from build123d import *

# Parameters (mm, degrees)
BOSS_EXTRUDE1_DEPTH = 20
BOSS_EXTRUDE2_REACH = 35.797


with BuildPart() as part:
    # Sketch1 → Boss-Extrude1 (new, symmetric)
    with BuildSketch(Plane(origin=(0, 0, 0), x_dir=(0, 0, -1), z_dir=(1, 0, 0))):
        Polygon((-8, 0), (-8, 17.5), (8, 17.5), (8, 0), (10.5, 0), (10.5, 20), (-10.5, 20), (-10.5, 0), align=None)
    extrude(amount=BOSS_EXTRUDE1_DEPTH, both=True)

    # Sketch2 → Boss-Extrude2 (add, up to next)
    with BuildSketch(Plane(origin=(0, 0, 8), x_dir=(-1, 0, 0), z_dir=(0, 0, -1)), mode=Mode.PRIVATE) as boss_extrude2_sk1:
        with BuildLine():
            Line((20, 17.5), (20, 20))
            Line((20, 20), (-20, 20))
            Line((-20, 20), (-20, 17.5))
            ThreePointArc((-20, 17.5), (0, 9.985297678), (20, 17.5))
        make_face()
    boss_extrude2_tool1 = extrude(boss_extrude2_sk1.sketch, amount=BOSS_EXTRUDE2_REACH, mode=Mode.PRIVATE) - part.part
    add(boss_extrude2_tool1.solids().sort_by_distance((0, 15.86208, 8))[0])


solid = part.part
Read the model definition and answer for the solid it produces. Units are mm, in the model's axes. Round coordinates to 2 decimals unless told otherwise and drop trailing zeros. Write each loop counter-clockwise with the first axis right and the second up, starting at its lowest first coordinate (ties: lowest second). Pieces come first, ordered by that corner, then holes.
Q1. Straight lines are drawn through the part: line 1 (Z direction, x = 7.5, y = 2); line 2 (X direction, y = 13.5, z = -6); line 3 (Y direction, x = 10, z = 3). For each, find the intervals that lie inside material, in ascending order.
Values:
line 1: z = -10.5 to -8, 8 to 10.5
line 2: x = -14.18 to 14.18
line 3: y = 11.68 to 20
Q2. Find section D-D on x = 3.5. Determine the outline of the cut face in (y, z), and give its area (3 significant figures).
Values:
outline: (0, -10.5) - (20, -10.5) - (20, 10.5) - (0, 10.5) - (0, 8) - (10.19, 8) - (10.19, -8) - (0, -8) - close
area: 257 mm2
Q3. The mould has two halves that part along X. Classify faces 1 (the face through (0, 7, -8)), 2 (the face through (20, 18, 1)), 3 (the face through (0.306, 9.987, 0.112)), 4 (the face through (-20, 18, 1)): released by +X, released by -X, zero draft, split by the parting line, or undercut.
Values:
face 1: zero draft
face 2: released by +X
face 3: split by the parting line
face 4: released by -X
Q4. Find section B-B on z = -5. Determine the outline of the cut face in (x, y), and give its area (3 significant figures).
Values:
outline: (-20, 17.5) arc R30.37 ccw to (20, 17.5) - (20, 20) - (-20, 20) - close
area: 306 mm2
Q5. Find section A-A on y = 2. Determine the outline of the cut face in (x, z).
Values:
outline: (-20, -10.5) - (20, -10.5) - (20, -8) - (-20, -8) - close; (-20, 8) - (20, 8) - (20, 10.5) - (-20, 10.5) - close
Q6. Find section C-C on y = 16.25. Determine the outline of the cut face in (x, z), and give its area (3 significant figures).
Values:
outline: (-20, -10.5) - (20, -10.5) - (20, -8) - (18.47, -8) - (18.47, 8) - (20, 8) - (20, 10.5) - (-20, 10.5) - (-20, 8) - (-18.47, 8) - (-18.47, -8) - (-20, -8) - close
area: 791 mm2
Q7. Flat-ended cylindrical pins translate along their axes: P1, Ø10, axis at y = 12, z = 0, coming from the -X side; P2, Ø8, axis at y = 12, z = 2.5, coming from the -X side. Find the tip coordinate at first contact, or state that the pin passes through.
Values:
P1: stops at x = -19.41
P2: stops at x = -18.14
